```python
from build123d import *

# Parameters (mm, degrees)
SKETCH1_R          = 6.05
SKETCH1_W          = 4.5
SKETCH1_H          = 4.5
EXTRUDE1_DEPTH     = 100
CUT_EXTRUDE1_DEPTH = 101
CIRPATTERN1_COUNT  = 2
CIRPATTERN1_ANGLE  = 90


with BuildPart() as part:
    # Sketch1 → Extrude1 (new body)
    with BuildSketch(Plane.XY):
        Polygon((13, 7.265685), (11.634315, 7.265685), (8.3, 3.931371213), (8.3, -3.931371213), (11.634315, -7.265685), (13, -7.265685), (13, -4), (15, -4), (15, -15), (4, -15), (4, -13), (7.265685, -13), (7.265685, -11.634315), (3.931371213, -8.3), (-3.931371213, -8.3), (-7.265685, -11.634315), (-7.265685, -13), (-4, -13), (-4, -15), (-15, -15), (-15, -4), (-13, -4), (-13, -7.265685), (-11.634315, -7.265685), (-8.3, -3.931371213), (-8.3, 3.931371213), (-11.634315, 7.265685), (-13, 7.265685), (-13, 4), (-15, 4), (-15, 9.399999971), (-11.93005553, 9.399999971), (-9.99999999, 10.299999926), (-9.99999999, 11.534231082), (-7.49999999, 12.69999986), (-7.49999999, 13.499999971), (-14.999999992, 13.499999971), (-14.999999992, 15), (14.99999999, 15), (14.99999999, 13.499999971), (7.49999999, 13.499999971), (7.49999999, 12.69999986), (9.99999999, 11.534231082), (9.99999999, 10.299999926), (11.93005553, 9.399999971), (15, 9.399999971), (15, 4), (13, 4), align=None)
        Circle(SKETCH1_R, mode=Mode.SUBTRACT)
        Polygon((-8.5, 10.5786251), (-8.5, 9.344394771), (-10.60849553, 8.361187544), (-7.423547516, 5.176238259), (-3.426503445, 8.376249899), (-2.600251667, 7.55), (2.600251667, 7.55), (3.426503445, 8.376249899), (7.423547516, 5.176238259), (10.60849553, 8.361187544), (8.5, 9.344394771), (8.5, 10.5786251), (6, 11.7443949), (6, 13.5), (-6, 13.5), (-6, 11.7443949), align=None, mode=Mode.SUBTRACT)
        with Locations((-11.25, -11.25)):
            Rectangle(SKETCH1_W, SKETCH1_H, mode=Mode.SUBTRACT)
        with Locations((11.25, -11.25)):
            Rectangle(SKETCH1_W, SKETCH1_H, mode=Mode.SUBTRACT)
    extrude(amount=-EXTRUDE1_DEPTH)

    # Sketch2 → Cut-Extrude1 (cut, through all)
    with BuildSketch(Plane.XY):
        Polygon((-11.25, -9), (-7.686853797, -5.436853797), (-5.436853797, -7.686853797), (-9, -11.25), align=None)
    cut_extrude1 = extrude(amount=-CUT_EXTRUDE1_DEPTH, mode=Mode.SUBTRACT)

    # CirPattern1: Cut-Extrude1 ×2 about axis
    cirpattern1_axis = Axis((0, 0, 0), (0, 0, 1))
    for i in range(1, CIRPATTERN1_COUNT):
        add(cut_extrude1.rotate(cirpattern1_axis, i * CIRPATTERN1_ANGLE / (CIRPATTERN1_COUNT - 1)), mode=Mode.SUBTRACT)


solid = part.part
```
Read the model definition and answer for the solid it produces. Units are mm, in the model's axes. A direction names the side the tool comes from. Give positions to 0.01 mm unless a question says otherwise; leave off trailing zeros. Order: outer loops, then holes, each group sorted by start corner. A loop starts at its lowest first (then second) coordinate and runs counter-clockwise, first axis right, second up.
(1) For a pull along X with two mould halves and no side action, classify faces 6 (the flat face through (15, -9, -49)), 7 (the flat face through (12, -9, -49)), 8 (the flat face through (10, -15, -49)), 9 (the flat face through (-9.04, 6.79, -49.3)) as released by +X, released by -X, zero draft, split by the parting line, or undercut.
(2) Given pin 1 (0.9 mm diameter, centred on y = 13, z = -61.5, fed in from +X), flat-ended and moving along its own axis, determine where the tip first touches the part or whether it passes through.
(3) Find section C-C (z = -46.5). Give the number of separate pieces and of enclosed holes in the cut face, plus the area to 3 significant figures.
(4) Straight lines are drawn through the part: L1, parallel to Y at x = 0, z = -60; L2, parallel to X at y = -12.25, z = -32; L3, parallel to Y at x = 12.75, z = -38. For each, find the intervals that lie inside material, in ascending order.
(5) Find section B-B (x = 0). Give the vertices of the cut face in (y, z).
(6) Find section A-A (y = 0). Give the vertices of the cut face in (x, z), plus the area to 3 significant figures.
(7) For faces 1 (the flat face through (-15, 7, -49)), 2 (the flat face through (-4, -14, -49)), 3 (the flat face through (-6, -13, -49)), 4 (the flat face through (14, -4, -49)), 5 (the flat face through (-9, -15, -49)), determine the directions among +Z, -Z, +X, -X, +Y, -Y from which every point of the face is accessible in a straight line to the end or side of a thin tool.
Result sheet:
1. face 6: released by +X
1. face 7: undercut
1. face 8: zero draft
1. face 9: undercut
2. pin 1: stops at x = 7.82
3. separate pieces: 1
3. enclosed holes: 4
3. area: 346 mm2
4. L1: y = -8.3 to -6.05, 6.05 to 7.55, 13.5 to 15
4. L2: x = -15 to -13.5, -9 to -7.27, 7.27 to 9, 13.5 to 15
4. L3: y = -15 to -13.5, -9 to -7.27, 7.27 to 9.4, 13.5 to 15
5. outline: (-8.3, -100) - (-6.05, -100) - (-6.05, 0) - (-8.3, 0) - close; (6.05, -100) - (7.55, -100) - (7.55, 0) - (6.05, 0) - close; (13.5, -100) - (15, -100) - (15, 0) - (13.5, 0) - close
6. outline: (-8.3, -100) - (-6.05, -100) - (-6.05, 0) - (-8.3, 0) - close; (6.05, -100) - (8.3, -100) - (8.3, 0) - (6.05, 0) - close
6. area: 450 mm2
7. face 1: +Z, -Z, -X, +Y, -Y
7. face 2: +Z, -Z, -Y
7. face 3: +Z, -Z
7. face 4: +Z, -Z, +X
7. face 5: +Z, -Z, +X, -X, -Y
